```python
from build123d import *

# Parameters (mm, degrees)
SKETCH1_W                   = 6.35
SKETCH1_H                   = 44.45
BOSS_EXTRUDE1_DEPTH         = 457.2
FILLET1_R                   = 6.35
F_1_4_0_25_DIAMETER_HOLE1_D = 6.35
LPATTERN1_COUNT             = 4
LPATTERN1_PITCH             = 114.3
F_1_4_0_25_DIAMETER_HOLE2_D = 6.35
LPATTERN2_COUNT             = 4
LPATTERN2_PITCH             = 114.3


with BuildPart() as part:
    # Sketch1 → Boss-Extrude1 (new body)
    with BuildSketch(Plane.XY):
        with Locations((-26.434360713, 1.221912767)):
            Rectangle(SKETCH1_W, SKETCH1_H)
        Polygon((-23.259360713, -21.003087233), (-29.609360713, -21.003087233), (-29.609360713, -27.353087233), (21.190639287, -27.353087233), (21.190639287, -21.003087233), align=None)
    extrude(amount=BOSS_EXTRUDE1_DEPTH)

    # Fillet1
    fillet1_edges = [part.edges().sort_by_distance(p)[0] for p in [
        (-23.259360713, -21.003087233, 228.6),
    ]]
    fillet(fillet1_edges, radius=FILLET1_R)

    # 1/4 (0.25) Diameter Hole1 (through all)
    with Locations(Plane.XZ.offset(27.353087233)):
        with Locations((-4.209360713, 400.05)):
            f_1_4_0_25_diameter_hole1 = Hole(F_1_4_0_25_DIAMETER_HOLE1_D / 2)

    # LPattern1: 1/4 (0.25) Diameter Hole1 ×4
    with Locations(*[(0, 0, -i * LPATTERN1_PITCH) for i in range(1, LPATTERN1_COUNT)]):
        add(f_1_4_0_25_diameter_hole1, mode=Mode.SUBTRACT)

    # 1/4 (0.25) Diameter Hole2 (through all)
    with Locations(Plane.ZY.offset(29.609360713)):
        with Locations((400.05, -1.953087233)):
            f_1_4_0_25_diameter_hole2 = Hole(F_1_4_0_25_DIAMETER_HOLE2_D / 2)

    # LPattern2: 1/4 (0.25) Diameter Hole2 ×4
    with Locations(*[(0, 0, -i * LPATTERN2_PITCH) for i in range(1, LPATTERN2_COUNT)]):
        add(f_1_4_0_25_diameter_hole2, mode=Mode.SUBTRACT)


solid = part.part
```
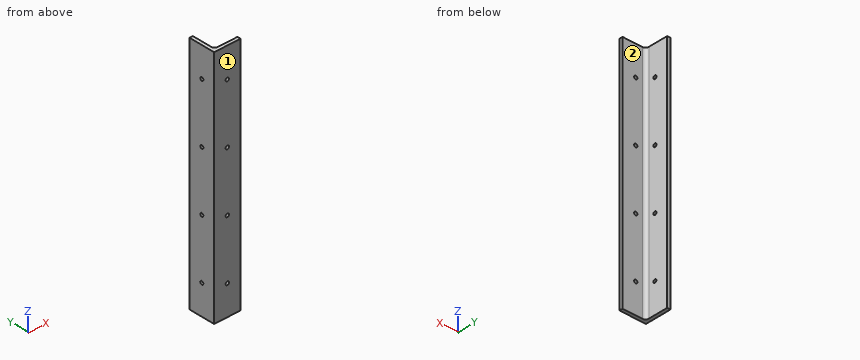
The model under review builds one solid part; all positions refer to its coordinate system, in mm. Face numbers are marked on the shaded views. A direction names the side the tool comes from. Round coordinates to 2 decimals unless told otherwise and drop trailing zeros. Order: outer loops, then holes, each group sorted by start corner. A loop starts at its lowest first (then second) coordinate and runs counter-clockwise, first axis right, second up. Notation, with made-up numbers: (49.5, 35) -> (71.5, 35) arc R29 ccw to (71.5, 72) -> close; hole circle Ø8 at (0, 34). An arc over 180 degrees is marked (long way). Use a Markdown table: item, result.
Q1. For line 1 (Y direction, x = -26, z = 57); line 2 (X direction, y = -24, z = 400.05); line 3 (Y direction, x = -15, z = 111.5), list the stretches that pass through material, from the lowest coordinate up.
Values:
| item | result |
|---|---|
| line 1 | y = -27.35 to -5.12, 1.22 to 23.45 |
| line 2 | x = -29.61 to -7.38, -1.03 to 21.19 |
| line 3 | y = -27.35 to -21 |
Q2. We need section A-A on z = 231. Write out the cut boundary in (x, y), then the cut area to 3 significant figures.
Values:
| item | result |
|---|---|
| outline | (-29.61, -27.35) -> (21.19, -27.35) -> (21.19, -21) -> (-16.91, -21) arc R6.35 cw to (-23.26, -14.65) -> (-23.26, 23.45) -> (-29.61, 23.45) -> close |
| area | 613 mm^2 |
Q3. We need section B-B on y = 15.5. Write out the cut boundary in (x, z).
Values:
| item | result |
|---|---|
| outline | (-29.61, 0) -> (-23.26, 0) -> (-23.26, 457.2) -> (-29.61, 457.2) -> close |
Q4. Clearance check with flat-ended pins moving along their axes: P1, Ø11.5, axis at x = -3, z = 125, coming from the +Y side; P2, Ø10, axis at y = -1.95, z = 285.75, coming from the -X side; P3, Ø5.5, axis at x = -4.21, z = 57.15, coming from the +Y side; P4, Ø3, axis at y = 3.5, z = 172, coming from the +X side. State where each tip first meets the part, or that it passes through.
Values:
| item | result |
|---|---|
| P1 | stops at y = -21 |
| P2 | stops at x = -29.61 |
| P3 | passes through |
| P4 | stops at x = -23.26 |
Q5. We need section C-C on x = -13. Write out the cut boundary in (y, z).
Values:
| item | result |
|---|---|
| outline | (-27.35, 0) -> (-21, 0) -> (-21, 457.2) -> (-27.35, 457.2) -> close |
Q6. Tool access review of the marked faces 1 and 2: name each direction out of +Z, -Z, +X, -X, +Y, -Y from which nothing blocks a thin tool from reaching the whole face with its end or side.
Values:
| item | result |
|---|---|
| face 1 | +Z, -Z, +X, -X, -Y |
| face 2 | +Z, -Z, +X, +Y |
